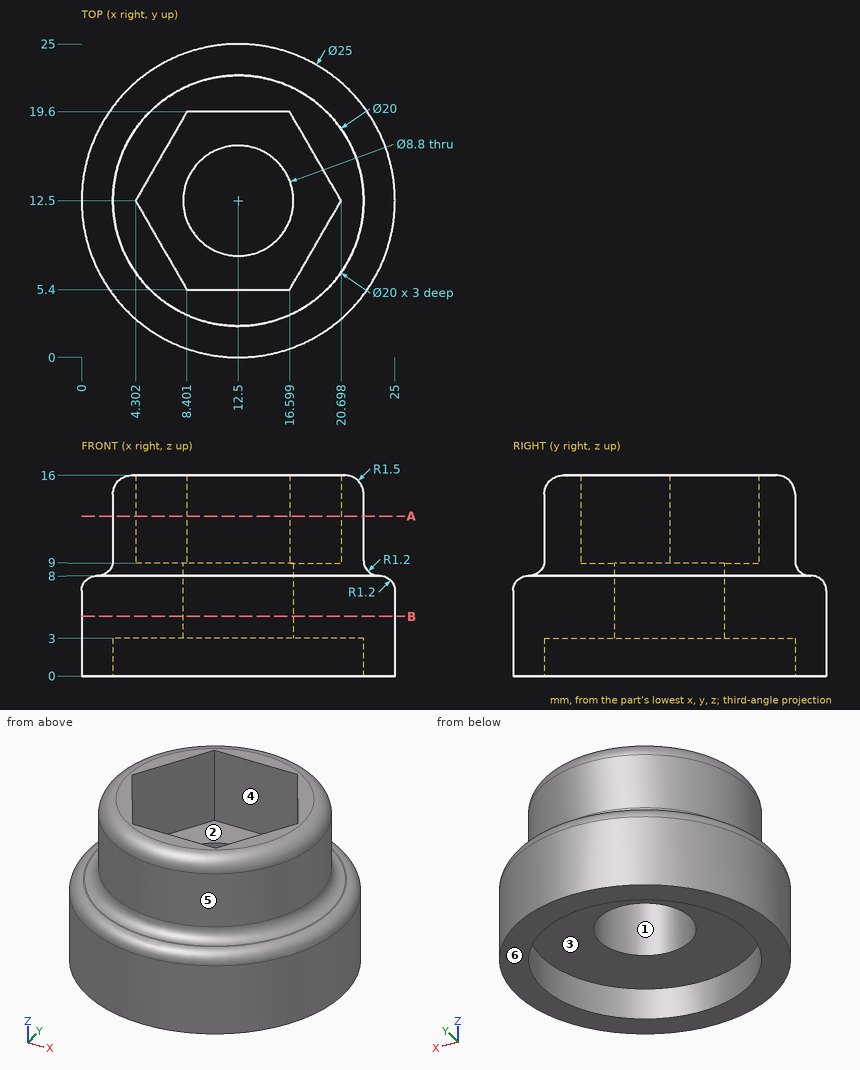
Drawing for the job (mm, zero at the part's lowest x, y, z). A direction names the side the tool comes from. Give positions to 0.01 mm unless a question says otherwise; leave off trailing zeros. Order: outer loops, then holes, each group sorted by start corner. A loop starts at its lowest first (then second) coordinate and runs counter-clockwise, first axis right, second up. Notation, with made-up numbers: M -33.75,3.25 L -16.75,3.25 A7 cw -16.75,14.25 Z; hole C 80,33 d3. An arc over 180 degrees is marked long. Put each result on its own line as item: value.
Item 1: Two-plate mould, pull along Y, no slides. Class the marked faces 4, 5 and 6: +Y half, -Y half, draft (parallel to the pull), parting line (faces both ways), or undercut.
From the geometry:
face 4: undercut
face 5: parting line
face 6: draft
Item 2: Probe line 1 (Y direction, x = 12.5, z = 6.4); line 2 (Y direction, x = 12.5, z = 1.1); line 3 (Z direction, x = 17.75, y = 14.75). List the from-to ranges inside material, lowest first. Write a range as [from, to].
From the geometry:
line 1: y = [0, 8.1], [16.9, 25]
line 2: y = [0, 2.5], [22.5, 25]
line 3: z = [3, 9]
Item 3: Slice it at B-B, the plane z = 4.75. Write the cut outline in (x, y).
From the geometry:
outline: C 12.5,12.5 d25; hole C 12.5,12.5 d8.8
Item 4: Flat gauge pins, fed straight in: pin 1 Ø7.5 at (x, z) = (12, 11) entering from -Y; pin 2 Ø3 at (y, z) = (8.5, 8.5) entering from +X; pin 3 Ø6 at (x, z) = (8, 10) entering from -Y; pin 4 Ø1.5 at (x, y) = (11, 11.5) entering from +Z. Where does each tip first touch, or does it go through?
From the geometry:
pin 1: stops at y = 0.09
pin 2: stops at x = 24.5
pin 3: stops at y = 0.53
pin 4: passes through
Item 5: 3-axis set-ups, long thin cutter, end or side, ignore diameter. For the marked faces 1, 2 and 3: which of +Z, -Z, +X, -X, +Y, -Y reach the whole face in a straight line?
From the geometry:
face 1: +Z, -Z
face 2: +Z
face 3: -Z
Item 6: Slice it at A-A, the plane z = 12.75. Write the cut outline in (x, y).
From the geometry:
outline: C 12.5,12.5 d20; hole M 4.3,12.5 L 8.4,5.4 L 16.6,5.4 L 20.7,12.5 L 16.6,19.6 L 8.4,19.6 Z
